Input: part model. Units: mm. Frame: model coordinates. Face numbers are marked on the shaded views. Round coordinates to 2 decimals unless told otherwise and drop trailing zeros. Order: outer loops, then holes, each group sorted by start corner. A loop starts at its lowest first (then second) coordinate and runs counter-clockwise, first axis right, second up. Notation, with made-up numbers: (12, -13) - (54, -13) arc R23 ccw to (54, -2) - close; hole circle Ø11 at (-5, 44.5). An arc over 180 degrees is marked (long way). One line per item, written item: value. Start each with the question number.
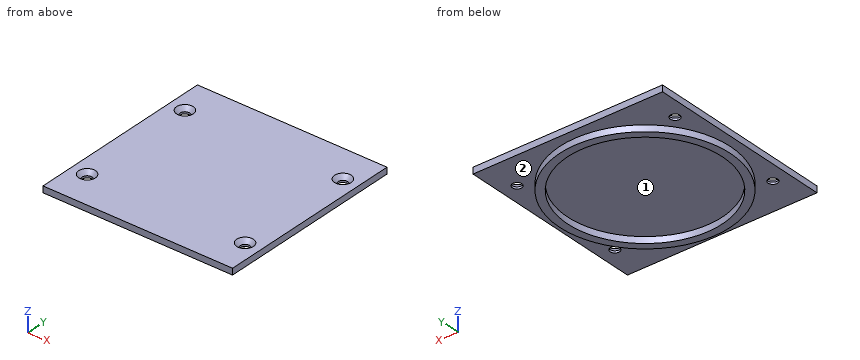
Autodesk Inventor part; units mm, degrees
ref_plane "YZ Plane" through (0, 0, 0) normal (1, 0, 0) x (0, 1, 0)
ref_plane "XZ Plane" through (0, 0, 0) normal (0, 1, 0) x (-1, 0, 0)
ref_plane "XY Plane" through (0, 0, 0) normal (0, 0, 1) x (1, 0, 0)
sketch "Boceto1" plane through (0, 0, 0) normal (0, 0, 1) x (1, 0, 0)
  line L0 (-30, 30) -> (30, 30)
  line L1 (30, 30) -> (30, -30)
  line L2 (30, -30) -> (-30, -30)
  line L3 (-30, -30) -> (-30, 30)
  line L4 (-30, 30) -> (30, -30) construction
  line L5 (30, 30) -> (-30, -30) construction
  point P0 (0, 0)
  dimension "d0" = 60
  dimension "d1" = 60
extrude "Extrusión1" add sketch "Boceto1" along normal blind 2
sketch "Boceto2" plane through (0, 0, 2) normal (0, 0, 1) x (1, 0, 0)
  circle A0 centre (-25, 19) radius 2.2
  circle A1 centre (-25, -19) radius 2.2
  circle A2 centre (25, -19) radius 2.2
  circle A3 centre (25, 19) radius 2.2
  point P0 (0, 0)
hole "Agujero1" at (25, 19, 2) at (-25, 19, 2) at (-25, -19, 2) at (25, -19, 2) direction (0, 0, -1) diameter 3 depth 2 countersink diameter 5.3 countersink angle 80
sketch "Boceto3" plane through (0, 0, 0) normal (0, 0, -1) x (-1, 0, 0)
  circle A0 centre (0, 0) radius 24.5
  circle A1 centre (0, 0) radius 27
  circle A2 centre (0, 0) radius 24.5
  circle A3 centre (0, 0) radius 27.5
  circle A4 centre (0, 0) radius 27.5
  point P0 (12.49, 24.5)
  point P1 (12.49, -24.5)
  dimension "d13" = 54
extrude "Extrusión2" add sketch "Boceto3" along normal blind 2 contours A1
properties part number "Tapa"
Item 1: Section query B-B on x = 0. Return loops of the section in (y, z).
Item 2: Line query: L1, parallel to Y at x = -25, z = 0.3; L2, parallel to X at y = -19, z = 0.2; L3, parallel to Y at x = 0, z = -0.8. Output: solid intervals per line, ascending.
Item 3: Section query A-A on y = 19. Return loops of the section in (x, z).
Item 4: First-contact query: pin 1 Ø4 at (x, y) = (21.5, -7) entering from -Z; pin 2 Ø5 at (x, y) = (-25, -19) entering from +Z; pin 3 Ø5 at (x, y) = (-14, -1) entering from -Z; pin 4 Ø4 at (x, y) = (-25, 19) entering from +Z. Flat tips, straight axial feed; report the tip coordinate or a pass-through.
Item 5: Pull-direction query (Y, two-part tool) for the marked faces 1 and 2; classes: released by +Y, released by -Y, zero draft, split by the parting line, or undercut.
Item 6: Section query D-D on z = -1.2. Return loops of the section in (x, y).
Geometry results:
1. outline: (-30, 0) - (-27, 0) - (-27, -2) - (-24.5, -2) - (-24.5, 0) - (24.5, 0) - (24.5, -2) - (27, -2) - (27, 0) - (30, 0) - (30, 2) - (-30, 2) - close
2. L1: y = -30 to -20.5, -17.5 to 17.5, 20.5 to 30
2. L2: x = -30 to -26.5, -23.5 to 23.5, 26.5 to 30
2. L3: y = -27 to -24.5, 24.5 to 27
3. outline: (-30, 0) - (-26.5, 0) - (-26.5, 0.63) - (-27.65, 2) - (-30, 2) - close; (-23.5, 0) - (-19.18, 0) - (-19.18, -2) - (-15.47, -2) - (-15.47, 0) - (15.47, 0) - (15.47, -2) - (19.18, -2) - (19.18, 0) - (23.5, 0) - (23.5, 0.63) - (22.35, 2) - (-22.35, 2) - (-23.5, 0.63) - close; (26.5, 0) - (30, 0) - (30, 2) - (27.65, 2) - (26.5, 0.63) - close
4. pin 1: stops at z = -2
4. pin 2: stops at z = 1.82
4. pin 3: stops at z = 0
4. pin 4: stops at z = 1.23
5. face 1: undercut
5. face 2: zero draft
6. outline: circle Ø54 at (0, 0); hole circle Ø49 at (0, 0)
